Check sheet for the modelled part. Datum: model origin and axes. Units: mm. A direction names the side the tool comes from. Coordinates: 2 decimals unless noted, no trailing zeros. Order: outer loops, then holes, each group sorted by start corner. A loop starts at its lowest first (then second) coordinate and runs counter-clockwise, first axis right, second up.
1. Cross-section at B-B (x = 36). Enter the section's corners in (y, z).
2. Cross-section at C-C (y = -1.5). Enter the section's corners in (x, z), then the cut area to 3 significant figures.
3. Set-up check for faces 1 (the flat face through (24, -14, 0)), 2 (the flat face through (52.04, -9.634, 0.501)): record each of +Z, -Z, +X, -X, +Y, -Y from which the full face is reachable in a straight line by a thin tool's end or side.
4. Cross-section at A-A (z = 0.5). Enter the section's corners in (x, y), then the cut area to 3 significant figures.
5. Thickness scan on line 1 (Y direction, x = -5, z = 0.9); line 2 (X direction, y = 0.5, z = 0.4); line 3 (X direction, y = 6.5, z = 0.3). Record the ranges inside material, lowest first.
6. Draft check along Y on faces 3 (the flat face through (24, -14, 1.016)), 4 (the cylindrical face through (53.02, 7.93, 0.52)). Enter one of: released by +Y, released by -Y, zero draft, split by the parting line, or undercut.
```python
from build123d import *

# Parameters (mm, degrees)
F1_DEPTH = 1.016
F2_R     = 5.08
F3_SIZE  = 5.08


with BuildPart() as f1:
    # F0 (on Top) → F1 (new body)
    with BuildSketch(Plane.XY):
        Polygon((57.084747, -19.829684), (57.084747, -12.209684), (54.544747, -12.209684), (-12.511253, -12.209684), (-15.051253, -12.209684), (-15.051253, -19.829684), align=None)
        Polygon((57.084747, -12.209684), (57.084747, 11.920316), (-15.051253, 11.920316), (-15.051253, -12.209684), (-12.511253, -12.209684), (-12.511253, 9.380316), (54.544747, 9.380316), (54.544747, -12.209684), align=None)
    extrude(amount=F1_DEPTH)

    # F2
    f2_edges = [f1.edges().sort_by_distance(p)[0] for p in [
        (-12.511253, 9.380316, 0.508),
        (54.544747, 9.380316, 0.508),
    ]]
    fillet(f2_edges, radius=F2_R)

    # F3
    f3_edges = [f1.edges().sort_by_distance(p)[0] for p in [
        (-12.511253, -12.209684, 0.508),
        (54.544747, -12.209684, 0.508),
    ]]
    chamfer(f3_edges, length=F3_SIZE)


solid = f1.part
```
Data:
1. outline: (-19.83, 0) - (-12.21, 0) - (-12.21, 1.02) - (-19.83, 1.02) - close; (9.38, 0) - (11.92, 0) - (11.92, 1.02) - (9.38, 1.02) - close
2. outline: (-15.05, 0) - (-12.51, 0) - (-12.51, 1.02) - (-15.05, 1.02) - close; (54.54, 0) - (57.08, 0) - (57.08, 1.02) - (54.54, 1.02) - close
2. area: 5.16 mm2
3. face 1: -Z, +X, -X, +Y, -Y
3. face 2: +Z, -Z
4. outline: (-15.05, -19.83) - (57.08, -19.83) - (57.08, 11.92) - (-15.05, 11.92) - close; hole (-12.51, -7.13) - (-7.43, -12.21) - (49.46, -12.21) - (54.54, -7.13) - (54.54, 4.3) arc R5.08 ccw to (49.46, 9.38) - (-7.43, 9.38) arc R5.08 ccw to (-12.51, 4.3) - close
4. area: 879 mm2
5. line 1: y = -19.83 to -12.21, 9.38 to 11.92
5. line 2: x = -15.05 to -12.51, 54.54 to 57.08
5. line 3: x = -15.05 to -12.01, 54.04 to 57.08
6. face 3: zero draft
6. face 4: undercut
